Read the model definition and answer for the solid it produces. Units are mm, in the model's axes. Face numbers are marked on the shaded views. A direction names the side the tool comes from. Give positions to 0.01 mm unless a question says otherwise; leave off trailing zeros. Write each loop counter-clockwise with the first axis right and the second up, starting at its lowest first coordinate (ties: lowest second). Pieces come first, ordered by that corner, then holes. Notation, with made-up numbers: (75, -28) - (98, -28) arc R18 ccw to (98, -15) - close; hole circle Ø3 at (75, -18). An arc over 180 degrees is marked (long way). Answer as CSV lines item,"result".
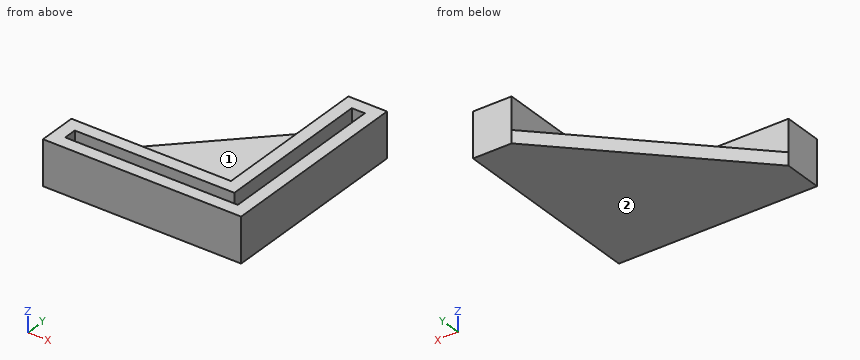
```python
from build123d import *

# Parameters (mm, degrees)
F0_W     = 0.82
F0_H     = 0.8
F0_W_2   = 0.8
F0_H_2   = 0.82
F1_DEPTH = 2
F2_DEPTH = 0.8


with BuildPart() as f1:
    # F0 (on Top) → F1 (new body)
    with BuildSketch(Plane.XY):
        Polygon((-10.41, 0.41), (-0.41, 0.41), (-0.41, 10.41), (0.41, 10.41), (0.41, 0.41), (1.21, 0.41), (1.21, 1.21), (1.21, 11.21), (-1.21, 11.21), (-1.21, 1.21), (-11.21, 1.21), (-11.21, -1.21), (-1.21, -1.21), (-0.41, -1.21), (-0.41, -0.41), (-10.41, -0.41), align=None)
        with Locations((0, -0.81)):
            Rectangle(F0_W, F0_H)
        with Locations((0.81, 0)):
            Rectangle(F0_W_2, F0_H_2)
        with Locations((0.81, -0.81)):
            Rectangle(F0_W_2, F0_H)
    extrude(amount=F1_DEPTH)

    # F0 (on Top) + F1_face (on face) → F2 (join)
    with BuildSketch(Plane.XY):
        Polygon((-1.21, 1.21), (-1.21, 11.21), (-11.21, 1.21), align=None)
        Polygon((-10.41, 0.41), (-0.41, 0.41), (-0.41, 10.41), (0.41, 10.41), (0.41, 0.41), (1.21, 0.41), (1.21, 1.21), (1.21, 11.21), (-1.21, 11.21), (-1.21, 1.21), (-11.21, 1.21), (-11.21, -1.21), (-1.21, -1.21), (-0.41, -1.21), (-0.41, -0.41), (-10.41, -0.41), align=None)
        Polygon((-0.41, 10.41), (-0.41, 0.41), (-10.41, 0.41), (-10.41, -0.41), (-0.41, -0.41), (0.41, -0.41), (0.41, 0.41), (0.41, 10.41), align=None)
        with Locations((0, -0.81)):
            Rectangle(F0_W, F0_H)
        with Locations((0.81, 0)):
            Rectangle(F0_W_2, F0_H_2)
        with Locations((0.81, -0.81)):
            Rectangle(F0_W_2, F0_H)
    with BuildSketch(Plane(origin=(-2.8485370052, 2.8485370052, 2), x_dir=(1, 0, 0), z_dir=(0, 0, 1))):
        Polygon((-8.3614629948, -4.0585370052), (4.0585370052, -4.0585370052), (4.0585370052, 8.3614629948), (1.6385370052, 8.3614629948), (1.6385370052, -1.6385370052), (-8.3614629948, -1.6385370052), align=None)
        Polygon((3.2585370052, 7.5614629948), (3.2585370052, -3.2585370052), (-7.5614629948, -3.2585370052), (-7.5614629948, -2.4385370052), (2.4385370052, -2.4385370052), (2.4385370052, 7.5614629948), align=None, mode=Mode.SUBTRACT)
    extrude(amount=-F2_DEPTH)


solid = f1.part
```
(1) Find the intervals of material crossed by L1, parallel to Y at x = 0, z = 1.85; L2, parallel to X at y = 5.5, z = 0.4; L3, parallel to Y at x = -0.5, z = 0.6, in increasing order.
Worked out:
L1,"y = -1.21 to -0.41, 10.41 to 11.21"
L2,"x = -1.21 to -0.41, 0.41 to 1.21"
L3,"y = -1.21 to -0.41, 0.41 to 11.21"
(2) Each of these flat-tipped pins is pushed along its axis until it touches: P1, Ø1, axis at y = 3, z = 1.5, coming from the -X side; P2, Ø4, axis at x = -8, y = 6.5, coming from the +Z side; P3, Ø1.6, axis at x = -2.5, z = 1, coming from the +Y side. Where does it stop, or does it pass through?
Worked out:
P1,"stops at x = -1.21"
P2,"stops at z = 0"
P3,"stops at y = 1.21"
(3) A cutting plane is placed at B-B (x = -1.75). Write down the section's boundary in (y, z), and give its area (3 significant figures).
Worked out:
outline,"(-1.21, -0.8) - (10.67, -0.8) - (10.67, 0) - (1.21, 0) - (1.21, 2) - (0.41, 2) - (0.41, 0) - (-0.41, 0) - (-0.41, 2) - (-1.21, 2) - close"
area,"12.7 mm^2"
(4) A cutting plane is placed at A-A (z = 0.4). Write down the section's boundary in (x, y).
Worked out:
outline,"(-11.21, -1.21) - (1.21, -1.21) - (1.21, 11.21) - (-1.21, 11.21) - (-1.21, 1.21) - (-11.21, 1.21) - close; hole (-10.41, -0.41) - (0.41, -0.41) - (0.41, 10.41) - (-0.41, 10.41) - (-0.41, 0.41) - (-10.41, 0.41) - close"
(5) A cutting plane is placed at D-D (y = 10.75). Write down the section's boundary in (x, z).
Worked out:
outline,"(-1.67, -0.8) - (1.21, -0.8) - (1.21, 2) - (-1.21, 2) - (-1.21, 0) - (-1.67, 0) - close"
(6) A cutting plane is placed at C-C (y = 5.25). Write down the section's boundary in (x, z), and give its area (3 significant figures).
Worked out:
outline,"(-7.17, -0.8) - (1.21, -0.8) - (1.21, 2) - (0.41, 2) - (0.41, 0) - (-0.41, 0) - (-0.41, 2) - (-1.21, 2) - (-1.21, 0) - (-7.17, 0) - close"
area,"9.90 mm^2"
(7) For the marked faces 1 and 2, determine the directions among +Z, -Z, +X, -X, +Y, -Y from which every point of the face is accessible in a straight line to the end or side of a thin tool.
Worked out:
face 1,"+Z, -X, +Y"
face 2,"-Z, +X, -X, +Y, -Y"
